Design review of the part built by this model. Coordinates are the model's own, in mm. A direction names the side the tool comes from. Round coordinates to 2 decimals unless told otherwise and drop trailing zeros. Write each loop counter-clockwise with the first axis right and the second up, starting at its lowest first coordinate (ties: lowest second). Pieces come first, ordered by that corner, then holes. Notation, with made-up numbers: M 72,25 L 104,25 A13 ccw 104,29 Z; hole C 79,35.25 d7. An arc over 180 degrees is marked long. One line per question, with ' | ' between items. Start each with the question number.
Item 1: Machinability: for faces 1 (the face through (5.72, 23.55, 11.7)), 2 (the face through (3, 6.411, 12)), 3 (the face through (3.15, 2.73, 0.09)), 4 (the face through (3, -10.099, 5)), 5 (the face through (0.63, 23.55, 11.7)), which of the approach directions +Z, -Z, +X, -X, +Y, -Y give a long, thin tool a straight path to every point of the face, cutting with its end or side? Answer none if there is none.
Item 2: Add section B-B, the plane x = 2.75. State the section outline as (y, z) points.
Item 3: Add section C-C, the plane z = 0.75. Give the number of separate pieces and of enclosed holes in the cut face, and give its area (3 significant figures).
Item 4: Add section A-A, the plane z = 14.25. State the section outline as (x, y) points.
Item 5: Insertion check: pin 1 Ø10 at (y, z) = (2.6, 4.41) entering from +X; pin 2 Ø8 at (y, z) = (-4.5, 6.5) entering from -X; pin 3 Ø1 at (x, y) = (2.5, 31) entering from +Z; pin 4 Ø3 at (y, z) = (2, 3.5) entering from -X. Each pin has a flat end and moves straight along its axis. Give the tip position at first contact, or say it passes through.
Item 6: For L1, parallel to Y at x = 0.5, z = 4.75; L2, parallel to Y at x = 4.75, z = 13; L3, parallel to Z at x = 2.5, y = 28.5, list the stretches that pass through material, from the lowest coordinate up.
Item 7: Draft analysis for pull direction Z (two halves, no side actions). For faces 6 (the face through (5.3, 28.13, -0.13)), 7 (the face through (3, 36, 17.105)), 8 (the face through (0.626, 7.055, 11.846)), 9 (the face through (5.3, 2.73, -0.13)), state which applies: released by +Z, released by -Z, zero draft, split by the parting line, or undercut.
```python
from build123d import *

# Parameters (mm, degrees)
F1_DEPTH = 6.35
F2_SIZE  = 1.27


# Not quite as in the source:
# - a feature names something its author has since deleted; it is built from what else it names


with BuildPart() as f1:
    # F0 (on Right) → F1 (new body)
    with BuildSketch(Plane.YZ):
        with BuildLine():
            Line((-10.0986241174, -8.2946426358), (40.7013758826, -8.2946426358))
            Line((40.7013758826, -8.2946426358), (40.7013758826, 17.1053573642))
            Line((40.7013758826, 17.1053573642), (31.8113758826, 17.1053573642))
            Line((31.8113758826, 17.1053573642), (31.8113758826, 6.4373573642))
            ThreePointArc((31.8113758826, 6.4373573642), (28.0013758826, 0.0873573642), (24.1913758826, 6.4373573642))
            Line((24.1913758826, 6.4373573642), (24.1913758826, 17.1053573642))
            Line((24.1913758826, 17.1053573642), (15.3013758826, 17.1053573642))
            Line((15.3013758826, 17.1053573642), (6.4113758826, 17.1053573642))
            Line((6.4113758826, 17.1053573642), (6.4113758826, 6.4373573642))
            ThreePointArc((6.4113758826, 6.4373573642), (2.6013758826, 0.0873573642), (-1.2086241174, 6.4373573642))
            Line((-1.2086241174, 6.4373573642), (-1.2086241174, 17.1053573642))
            Line((-1.2086241174, 17.1053573642), (-10.0986241174, 17.1053573642))
            Line((-10.0986241174, 17.1053573642), (-10.0986241174, -8.2946426358))
        make_face()
    extrude(amount=F1_DEPTH)

    # F2
    f2_edges = [f1.edges().sort_by_distance(p)[0] for p in [
        (6.35, -1.208624, 11.771357),
        (6.35, 2.601376, 0.087357),
        (6.35, 6.411376, 11.771357),
        (6.35, 24.191376, 11.771357),
        (6.35, 28.001376, 0.087357),
        (6.35, 31.811376, 11.771357),
        (0, 2.601376, 0.087357),
        (0, -1.208624, 11.771357),
        (0, 24.191376, 11.771357),
        (0, 28.001376, 0.087357),
        (0, 31.811376, 11.771357),
        (0, 6.411376, 11.771357),
    ]]
    chamfer(f2_edges, length=F2_SIZE)


solid = f1.part
```
Computed values:
1) face 1: +Z, +X | face 2: +Z, +X, -X | face 3: +X, -X | face 4: +Z, -Z, +X, -X, -Y | face 5: +Z, -X
2) outline: M -10.1,-8.29 L 40.7,-8.29 L 40.7,17.11 L 31.81,17.11 L 31.81,6.44 A4.32 cw long 24.19,6.44 L 24.19,17.11 L 6.41,17.11 L 6.41,6.44 A4.32 cw long -1.21,6.44 L -1.21,17.11 L -10.1,17.11 Z
3) separate pieces: 3 | enclosed holes: 0 | area: 254 mm^2
4) outline: M 0,-10.1 L 6.35,-10.1 L 6.35,-2.48 L 5.08,-1.21 L 1.27,-1.21 L 0,-2.48 Z; M 0,7.68 L 1.27,6.41 L 5.08,6.41 L 6.35,7.68 L 6.35,22.92 L 5.08,24.19 L 1.27,24.19 L 0,22.92 Z; M 0,33.08 L 1.27,31.81 L 5.08,31.81 L 6.35,33.08 L 6.35,40.7 L 0,40.7 Z
5) pin 1: stops at x = 5.77 | pin 2: stops at x = 0 | pin 3: stops at z = 1.87 | pin 4: passes through
6) L1: y = -10.1 to -2.47, 7.68 to 22.93, 33.08 to 40.7 | L2: y = -10.1 to -1.21, 6.41 to 24.19, 31.81 to 40.7 | L3: z = -8.29 to 0.12
7) face 6: undercut | face 7: released by +Z | face 8: zero draft | face 9: undercut
